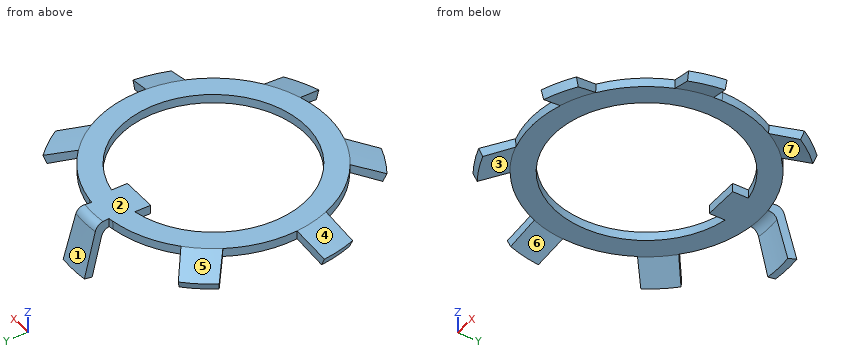
```python
from build123d import *

# Parameters (mm, degrees)
CUT_EXTRUDE2_DEPTH           = 24.379246777
CUT_EXTRUDE2_DEPTH_BACK      = 24.379246777
CUT_EXTRUDE4_DEPTH           = 10
CUT_EXTRUDE4_DRAFT           = 2
CUT_EXTRUDE4_PROFILE_2_DEPTH = 10
CUT_EXTRUDE4_PROFILE_2_DRAFT = 2
CUT_EXTRUDE4_PROFILE_3_DEPTH = 10
CUT_EXTRUDE4_PROFILE_3_DRAFT = 2
CUT_EXTRUDE4_PROFILE_4_DEPTH = 10
CUT_EXTRUDE4_PROFILE_4_DRAFT = 2
CUT_EXTRUDE4_PROFILE_5_DEPTH = 10
CUT_EXTRUDE4_PROFILE_5_DRAFT = 2
CUT_EXTRUDE4_PROFILE_6_DEPTH = 10
CUT_EXTRUDE4_PROFILE_6_DRAFT = 2
CUT_EXTRUDE4_PROFILE_7_DEPTH = 10
CUT_EXTRUDE4_PROFILE_7_DRAFT = 2
CUT_EXTRUDE4_PROFILE_8_DEPTH = 10
CUT_EXTRUDE4_PROFILE_8_DRAFT = 2
CUT_EXTRUDE4_PROFILE_9_DEPTH = 10
CUT_EXTRUDE4_PROFILE_9_DRAFT = 2
REVOLVE3_ANGLE               = 13
FILLET1_R                    = 1


with BuildPart() as part:
    # Sketch1 → Revolve1 (revolve)
    with BuildSketch(Plane(origin=(0, 0, 0), x_dir=(0, 0, -1), z_dir=(1, 0, 0)), mode=Mode.PRIVATE) as revolve1_sk:
        Polygon((-1, 7.5), (-1, 13), (0.529028795, 16.5), (1.445399555, 16.099669349), (0, 13), (0, 7.5), align=None)
    revolve(revolve1_sk.sketch.rotate(Axis((0, 0, 1), (0, 0, -1)), 90), axis=Axis((0, 0, 1), (0, 0, -1)))

    # Sketch2 → Cut-Extrude2 (cut, two sides: drawn at the far end of the back side and taken through both)
    with BuildSketch(Plane.XY.offset(-CUT_EXTRUDE2_DEPTH_BACK)):
        with BuildLine():
            Line((-2, 8.5), (-2, 10.307764064))
            ThreePointArc((-2, 10.307764064), (0, -10.5), (2, 10.307764064))
            Line((2, 10.307764064), (2, 8.5))
            Line((2, 8.5), (-2, 8.5))
        make_face()
    extrude(amount=CUT_EXTRUDE2_DEPTH + CUT_EXTRUDE2_DEPTH_BACK, mode=Mode.SUBTRACT)


with BuildPart() as cut_extrude4_tool:
    # Sketch3 → Cut-Extrude4 (with draft: the straight prism first)
    with BuildSketch(Plane.XY.offset(1)):
        with BuildLine():
            ThreePointArc((11.558121734, 11.775390524), (7.159081695, 14.86598632), (2, 16.378339354))
            Line((2, 16.378339354), (2, 12.845232579))
            ThreePointArc((2, 12.845232579), (5.640488609, 11.712595283), (8.795827626, 9.57253448))
            Line((8.795827626, 9.57253448), (11.558121734, 11.775390524))
        make_face()
    extrude(amount=-CUT_EXTRUDE4_DEPTH)
    # Cut-Extrude4: the draft: its side faces are tilted about the plane it starts from
    cut_extrude4_sides = [cut_extrude4_tool.faces().sort_by_distance(p)[0] for p in [
        (10.17697468, 10.673962502, -4),
        (7.159081695, 14.86598632, -4),
        (2, 14.611785966, -4),
        (5.640488609, 11.712595283, -4),
    ]]
    draft(cut_extrude4_sides, Plane.XY.offset(1), CUT_EXTRUDE4_DRAFT)


with BuildPart() as part_1:
    add(part.part)

    # Cut-Extrude4: cut by cut_extrude4_tool
    add(cut_extrude4_tool.part, mode=Mode.SUBTRACT)


with BuildPart() as cut_extrude4_profile_2_tool:
    # Sketch3 → Cut-Extrude4 profile 2 (with draft: the straight prism first)
    with BuildSketch(Plane.XY.offset(1)):
        with BuildLine():
            ThreePointArc((2, 16.378339354), (1.001848456, 16.469556754), (0, 16.5))
            Line((0, 16.5), (0, 13))
            ThreePointArc((0, 13), (1.00298965, 12.961250393), (2, 12.845232579))
            Line((2, 12.845232579), (2, 16.378339354))
        make_face()
    extrude(amount=-CUT_EXTRUDE4_PROFILE_2_DEPTH)
    # Cut-Extrude4 profile 2: the draft: its side faces are tilted about the plane it starts from
    cut_extrude4_profile_2_sides = [cut_extrude4_profile_2_tool.faces().sort_by_distance(p)[0] for p in [
        (2, 14.611785966, -4),
        (1.001848456, 16.469556754, -4),
        (0, 14.75, -4),
        (1.00298965, 12.961250393, -4),
    ]]
    draft(cut_extrude4_profile_2_sides, Plane.XY.offset(1), CUT_EXTRUDE4_PROFILE_2_DRAFT)


with BuildPart() as part_2:
    add(part_1.part)

    # Cut-Extrude4 profile 2: cut by cut_extrude4_profile_2_tool
    add(cut_extrude4_profile_2_tool.part, mode=Mode.SUBTRACT)


with BuildPart() as cut_extrude4_profile_3_tool:
    # Sketch3 → Cut-Extrude4 profile 3 (with draft: the straight prism first)
    with BuildSketch(Plane.XY.offset(1)):
        with BuildLine():
            Line((0, 13), (0, 16.5))
            ThreePointArc((0, 16.5), (-1.001848456, 16.469556754), (-2, 16.378339354))
            Line((-2, 16.378339354), (-2, 12.845232579))
            ThreePointArc((-2, 12.845232579), (-1.00298965, 12.961250393), (0, 13))
        make_face()
    extrude(amount=-CUT_EXTRUDE4_PROFILE_3_DEPTH)
    # Cut-Extrude4 profile 3: the draft: its side faces are tilted about the plane it starts from
    cut_extrude4_profile_3_sides = [cut_extrude4_profile_3_tool.faces().sort_by_distance(p)[0] for p in [
        (-1.00298965, 12.961250393, -4),
        (0, 14.75, -4),
        (-1.001848456, 16.469556754, -4),
        (-2, 14.611785966, -4),
    ]]
    draft(cut_extrude4_profile_3_sides, Plane.XY.offset(1), CUT_EXTRUDE4_PROFILE_3_DRAFT)


with BuildPart() as part_3:
    add(part_2.part)

    # Cut-Extrude4 profile 3: cut by cut_extrude4_profile_3_tool
    add(cut_extrude4_profile_3_tool.part, mode=Mode.SUBTRACT)


with BuildPart() as cut_extrude4_profile_4_tool:
    # Sketch3 → Cut-Extrude4 profile 4 (with draft: the straight prism first)
    with BuildSketch(Plane.XY.offset(1)):
        with BuildLine():
            Line((-2, 12.845232579), (-2, 16.378339354))
            ThreePointArc((-2, 16.378339354), (-7.159081695, 14.86598632), (-11.558121734, 11.775390524))
            Line((-11.558121734, 11.775390524), (-8.795827626, 9.57253448))
            ThreePointArc((-8.795827626, 9.57253448), (-5.640488609, 11.712595283), (-2, 12.845232579))
        make_face()
    extrude(amount=-CUT_EXTRUDE4_PROFILE_4_DEPTH)
    # Cut-Extrude4 profile 4: the draft: its side faces are tilted about the plane it starts from
    cut_extrude4_profile_4_sides = [cut_extrude4_profile_4_tool.faces().sort_by_distance(p)[0] for p in [
        (-10.17697468, 10.673962502, -4),
        (-5.640488609, 11.712595283, -4),
        (-2, 14.611785966, -4),
        (-7.159081695, 14.86598632, -4),
    ]]
    draft(cut_extrude4_profile_4_sides, Plane.XY.offset(1), CUT_EXTRUDE4_PROFILE_4_DRAFT)


with BuildPart() as part_4:
    add(part_3.part)

    # Cut-Extrude4 profile 4: cut by cut_extrude4_profile_4_tool
    add(cut_extrude4_profile_4_tool.part, mode=Mode.SUBTRACT)


with BuildPart() as cut_extrude4_profile_5_tool:
    # Sketch3 → Cut-Extrude4 profile 5 (with draft: the straight prism first)
    with BuildSketch(Plane.XY.offset(1)):
        with BuildLine():
            ThreePointArc((8.908232855, -13.888606388), (12.900219461, -10.287581731), (15.522658324, -5.594379194))
            Line((15.522658324, -5.594379194), (12.078133911, -4.808188975))
            ThreePointArc((12.078133911, -4.808188975), (10.163809272, -8.105367424), (7.375275277, -10.705387176))
            Line((7.375275277, -10.705387176), (8.908232855, -13.888606388))
        make_face()
    extrude(amount=-CUT_EXTRUDE4_PROFILE_5_DEPTH)
    # Cut-Extrude4 profile 5: the draft: its side faces are tilted about the plane it starts from
    cut_extrude4_profile_5_sides = [cut_extrude4_profile_5_tool.faces().sort_by_distance(p)[0] for p in [
        (12.900219461, -10.287581731, -4),
        (13.800396118, -5.201284084, -4),
        (10.163809272, -8.105367424, -4),
        (8.141754066, -12.296996782, -4),
    ]]
    draft(cut_extrude4_profile_5_sides, Plane.XY.offset(1), CUT_EXTRUDE4_PROFILE_5_DRAFT)


with BuildPart() as part_5:
    add(part_4.part)

    # Cut-Extrude4 profile 5: cut by cut_extrude4_profile_5_tool
    add(cut_extrude4_profile_5_tool.part, mode=Mode.SUBTRACT)


with BuildPart() as cut_extrude4_profile_6_tool:
    # Sketch3 → Cut-Extrude4 profile 6 (with draft: the straight prism first)
    with BuildSketch(Plane.XY.offset(1)):
        with BuildLine():
            Line((-3.771399805, -12.440922133), (-5.304357384, -15.624141344))
            ThreePointArc((-5.304357384, -15.624141344), (0, -16.5), (5.304357384, -15.624141344))
            Line((5.304357384, -15.624141344), (3.771399805, -12.440922133))
            ThreePointArc((3.771399805, -12.440922133), (0, -13), (-3.771399805, -12.440922133))
        make_face()
    extrude(amount=-CUT_EXTRUDE4_PROFILE_6_DEPTH)
    # Cut-Extrude4 profile 6: the draft: its side faces are tilted about the plane it starts from
    cut_extrude4_profile_6_sides = [cut_extrude4_profile_6_tool.faces().sort_by_distance(p)[0] for p in [
        (0, -16.5, -4),
        (4.537878594, -14.032531738, -4),
        (0, -13, -4),
        (-4.537878594, -14.032531738, -4),
    ]]
    draft(cut_extrude4_profile_6_sides, Plane.XY.offset(1), CUT_EXTRUDE4_PROFILE_6_DRAFT)


with BuildPart() as part_6:
    add(part_5.part)

    # Cut-Extrude4 profile 6: cut by cut_extrude4_profile_6_tool
    add(cut_extrude4_profile_6_tool.part, mode=Mode.SUBTRACT)


with BuildPart() as cut_extrude4_profile_7_tool:
    # Sketch3 → Cut-Extrude4 profile 7 (with draft: the straight prism first)
    with BuildSketch(Plane.XY.offset(1)):
        with BuildLine():
            Line((-12.078133911, -4.808188975), (-15.522658324, -5.594379194))
            ThreePointArc((-15.522658324, -5.594379194), (-12.900219461, -10.287581731), (-8.908232855, -13.888606388))
            Line((-8.908232855, -13.888606388), (-7.375275277, -10.705387176))
            ThreePointArc((-7.375275277, -10.705387176), (-10.163809272, -8.105367424), (-12.078133911, -4.808188975))
        make_face()
    extrude(amount=-CUT_EXTRUDE4_PROFILE_7_DEPTH)
    # Cut-Extrude4 profile 7: the draft: its side faces are tilted about the plane it starts from
    cut_extrude4_profile_7_sides = [cut_extrude4_profile_7_tool.faces().sort_by_distance(p)[0] for p in [
        (-13.800396118, -5.201284084, -4),
        (-12.900219461, -10.287581731, -4),
        (-8.141754066, -12.296996782, -4),
        (-10.163809272, -8.105367424, -4),
    ]]
    draft(cut_extrude4_profile_7_sides, Plane.XY.offset(1), CUT_EXTRUDE4_PROFILE_7_DRAFT)


with BuildPart() as part_7:
    add(part_6.part)

    # Cut-Extrude4 profile 7: cut by cut_extrude4_profile_7_tool
    add(cut_extrude4_profile_7_tool.part, mode=Mode.SUBTRACT)


with BuildPart() as cut_extrude4_profile_8_tool:
    # Sketch3 → Cut-Extrude4 profile 8 (with draft: the straight prism first)
    with BuildSketch(Plane.XY.offset(1)):
        with BuildLine():
            ThreePointArc((16.5, 0), (15.876229646, 4.493921699), (14.052080941, 8.648064594))
            Line((14.052080941, 8.648064594), (11.289786833, 6.44520855))
            ThreePointArc((11.289786833, 6.44520855), (12.565174667, 3.33412441), (13, 0))
            ThreePointArc((13, 0), (12.992051982, -0.454516548), (12.968217647, -0.908477326))
            Line((12.968217647, -0.908477326), (16.412742059, -1.694667545))
            ThreePointArc((16.412742059, -1.694667545), (16.478171075, -0.848456251), (16.5, 0))
        make_face()
    extrude(amount=-CUT_EXTRUDE4_PROFILE_8_DEPTH)
    # Cut-Extrude4 profile 8: the draft: its side faces are tilted about the plane it starts from
    cut_extrude4_profile_8_sides = [cut_extrude4_profile_8_tool.faces().sort_by_distance(p)[0] for p in [
        (16.086310551, 3.67159541, -4),
        (12.674062858, 2.892772141, -4),
        (12.670933887, 7.546636572, -4),
        (14.690479853, -1.301572436, -4),
    ]]
    draft(cut_extrude4_profile_8_sides, Plane.XY.offset(1), CUT_EXTRUDE4_PROFILE_8_DRAFT)


with BuildPart() as part_8:
    add(part_7.part)

    # Cut-Extrude4 profile 8: cut by cut_extrude4_profile_8_tool
    add(cut_extrude4_profile_8_tool.part, mode=Mode.SUBTRACT)


with BuildPart() as cut_extrude4_profile_9_tool:
    # Sketch3 → Cut-Extrude4 profile 9 (with draft: the straight prism first)
    with BuildSketch(Plane.XY.offset(1)):
        with BuildLine():
            Line((-11.289786833, 6.44520855), (-14.052080941, 8.648064594))
            ThreePointArc((-14.052080941, 8.648064594), (-16.086310551, 3.67159541), (-16.412742059, -1.694667545))
            Line((-16.412742059, -1.694667545), (-12.968217647, -0.908477326))
            ThreePointArc((-12.968217647, -0.908477326), (-12.674062858, 2.892772141), (-11.289786833, 6.44520855))
        make_face()
    extrude(amount=-CUT_EXTRUDE4_PROFILE_9_DEPTH)
    # Cut-Extrude4 profile 9: the draft: its side faces are tilted about the plane it starts from
    cut_extrude4_profile_9_sides = [cut_extrude4_profile_9_tool.faces().sort_by_distance(p)[0] for p in [
        (-16.086310551, 3.67159541, -4),
        (-14.690479853, -1.301572436, -4),
        (-12.674062858, 2.892772141, -4),
        (-12.670933887, 7.546636572, -4),
    ]]
    draft(cut_extrude4_profile_9_sides, Plane.XY.offset(1), CUT_EXTRUDE4_PROFILE_9_DRAFT)


with BuildPart() as part_9:
    add(part_8.part)

    # Cut-Extrude4 profile 9: cut by cut_extrude4_profile_9_tool
    add(cut_extrude4_profile_9_tool.part, mode=Mode.SUBTRACT)

    # Sketch4 → Revolve3 (revolve, symmetric)
    with BuildSketch(Plane(origin=(0, 0, 0), x_dir=(0, 0, -1), z_dir=(1, 0, 0))) as revolve3_sk:
        Polygon((-1, 10), (-1, 14.5), (4.795554958, 16.052914271), (5.054374003, 15.086988444), (0, 13.732673012), (0, 10), align=None)
    revolve(axis=Axis((0, 0, 1), (0, 0, -1)), revolution_arc=REVOLVE3_ANGLE / 2)
    revolve(revolve3_sk.sketch, axis=Axis((0, 0, 1), (0, 0, 1)), revolution_arc=REVOLVE3_ANGLE / 2)

    # Fillet1
    fillet1_edges = [part_9.edges().sort_by_distance(p)[0] for p in [
        (0, 14.5, 1),
        (0, 13.732673012, 0),
    ]]
    fillet(fillet1_edges, radius=FILLET1_R)


solid = part_9.part
```
Work out the finished part from the listing and answer in its coordinate system (mm). Face numbers are marked on the shaded views. A direction names the side the tool comes from. Round coordinates to 2 decimals unless told otherwise and drop trailing zeros. Write each loop counter-clockwise with the first axis right and the second up, starting at its lowest first coordinate (ties: lowest second). Pieces come first, ordered by that corner, then holes.
1) A cutting plane is placed at A-A on x = 0. Determine the outline of the cut face in (y, z).
2) Which of the six approach directions +Z, -Z, +X, -X, +Y, -Y give full straight-line access (tool end or side, diameter ignored) to the marked faces 5, 6 and 7?
3) Consider probe 1 along Z at (x, y) = (-11, 3); probe 2 along X at (y, z) = (0, 0.8); probe 3 along Y at (x, z) = (0, 0.5). Determine where each line is inside the solid, lowest interval first.
4) A cutting plane is placed at C-C on z = -4.25. Determine the outline of the cut face in (x, y).
5) Flat-ended cylindrical pins translate along their axes: P1, Ø4, axis at x = -7.5, y = 4.5, coming from the -Z side; P2, Ø1.5, axis at x = -2, y = -10, coming from the +Z side; P3, Ø3, axis at x = -12, z = -1, coming from the -Y side. Find the tip coordinate at first contact, or state that the pin passes through.
6) A cutting plane is placed at B-B on y = 11. Give the number of separate pieces and of enclosed holes in the cut face, and give its area (3 significant figures).
7) Determine the mould class of the marked faces 1, 2, 3 and 4 for opening direction X: pulls with the +X half, pulls with the -X half, needs draft (parallel to the pull), parting line crosses it, or undercut.
Entries:
1. outline: (-13, 1) - (-12.97, 0) - (-10.5, 0) - (-10.5, 1) - close; (8.5, 0) - (12.97, 0) arc R1 cw to (13.93, -0.74) - (15.09, -5.05) - (16.05, -4.8) - (14.7, 0.26) arc R1 ccw to (13.73, 1) - (8.5, 1) - close
2. face 5: +Z, -X, +Y
2. face 6: -Z
2. face 7: -Z, -Y
3. probe 1: z = 0 to 1
3. probe 2: x = -12.99 to -10.5, 10.5 to 12.99
3. probe 3: y = -12.98 to -10.5, 8.5 to 14.6
4. outline: (-1.8, 15.8) - (-1.68, 14.78) arc R14.87 cw to (1.68, 14.78) - (1.8, 15.8) arc R15.91 ccw to start
5. P1: stops at z = 0
5. P2: stops at z = 1
5. P3: stops at y = -7.05
6. separate pieces: 3
6. enclosed holes: 0
6. area: 16.7 mm2
7. face 1: parting line crosses it
7. face 2: needs draft
7. face 3: undercut
7. face 4: pulls with the -X half
